Geometry check sheet. Reference: the model listing, model coordinates, mm. Coordinates: 2 decimals unless noted, no trailing zeros. Write each loop counter-clockwise with the first axis right and the second up, starting at its lowest first coordinate (ties: lowest second). Pieces come first, ordered by that corner, then holes. Notation, with made-up numbers: M 49,17 L 85,17 A22 cw 85,54 Z; hole C -35.5,13 d11. An arc over 180 degrees is marked long. Put each result on its own line as item: value. Start each with the question number.
1) Scan lines: line 1 along X through (y, z) = (0, -7.15); line 2 along Z through (x, y) = (132, -2.75); line 3 along X through (y, z) = (6.75, -0.25). Record each from-to range of solid material in increasing order.
2) Gauge pin test, flat ends, axial feed: pin 1 (5 mm diameter, centred on y = -7.5, z = -3.5, fed in from -X); pin 2 (10 mm diameter, centred on x = 903, y = 5.5, fed in from +Z); pin 3 (3 mm diameter, centred on x = 43.5, y = 1, fed in from +Z). Record the tip position at first contact, or that the pin passes through.
3) Cross-section at A-A on x = 508. Record the cut outline in (y, z).
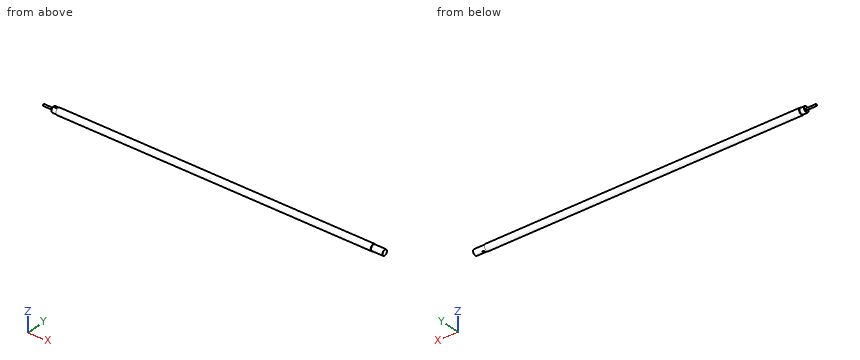
from build123d import *

# Parameters (mm, degrees)
CUT_EXTRUDE_1_DEPTH = 1.2
SKETCH_5_R          = 4
CUT_EXTRUDE_2_DEPTH = 5


with BuildPart() as part:
    # Sketch 1 → Revolve 1 (revolve)
    with BuildSketch(Plane.XY, mode=Mode.PRIVATE) as revolve_1_sk:
        with BuildLine():
            Line((51, 10.2), (51, 10.5))
            Line((51, 10.5), (51.5, 11))
            Line((51.5, 11), (1144.5, 11))
            Line((1144.5, 11), (1145, 10.5))
            Line((1145, 10.5), (1145, 10.2))
            ThreePointArc((1145, 10.2), (1145.058578644, 10.058578644), (1145.2, 10))
            Line((1145.2, 10), (1184.5, 10))
            Line((1184.5, 10), (1185, 9.5))
            Line((1185, 9.5), (1185, 0))
            Line((1185, 0), (720.314175827, 0))
            Line((720.314175827, 0), (0, 0))
            Line((0, 0), (0, 2.5))
            Line((0, 2.5), (0.5, 3))
            Line((0.5, 3), (34.5, 3))
            ThreePointArc((34.5, 3), (34.853553391, 3.146446609), (35, 3.5))
            Line((35, 3.5), (35, 9.5))
            Line((35, 9.5), (35.5, 10))
            Line((35.5, 10), (50.8, 10))
            ThreePointArc((50.8, 10), (50.941421356, 10.058578644), (51, 10.2))
        make_face()
    revolve(revolve_1_sk.sketch.rotate(Axis((0, 0, 0), (1, 0, 0)), 90), axis=Axis((0, 0, 0), (1, 0, 0)))

    # Sketch 3 → Cut-Extrude 1 (cut)
    with BuildSketch(Plane.XY.offset(10)):
        with BuildLine():
            Line((39, 3), (47, 3))
            ThreePointArc((47, 3), (50, 0), (47, -3))
            Line((47, -3), (39, -3))
            ThreePointArc((39, -3), (36, 0), (39, 3))
        make_face()
    extrude(amount=-CUT_EXTRUDE_1_DEPTH, mode=Mode.SUBTRACT)

    # Sketch 5 → Cut-Extrude 2 (cut)
    with BuildSketch(Plane(origin=(0, 0, -10), x_dir=(-1, 0, 0), z_dir=(0, 0, -1))):
        with Locations((-1155, 0)):
            Circle(SKETCH_5_R)
    extrude(amount=-CUT_EXTRUDE_2_DEPTH, mode=Mode.SUBTRACT)


solid = part.part
Answer key:
1. line 1: x = 35 to 1151, 1159 to 1185
1. line 2: z = -10.65 to 10.65
1. line 3: x = 35 to 1185
2. pin 1: stops at x = 35
2. pin 2: stops at z = 10.99
2. pin 3: stops at z = 8.8
3. outline: C 0,0 d22
